```python
from build123d import *

# Parameters (mm, degrees)
BOSS_EXTRUDE1_DEPTH = 3
SKETCH2_R           = 1.55
CUT_EXTRUDE1_DEPTH  = 356.878676658
BOSS_EXTRUDE3_START = -6
SKETCH3_R           = 1.55
BOSS_EXTRUDE3_DEPTH = 6


with BuildPart() as part:
    # Sketch1 → Boss-Extrude1 (new body)
    with BuildSketch(Plane(origin=(0, 0, 0), x_dir=(1, 0, 0), z_dir=(0, 1, 0))):
        Polygon((5.02071, 249.35), (4.05, 248.379), (4.05, 235), (4.04962, 234.998), (4.04981, 234.996), (4.04812, 234.989), (4.04698, 234.983), (4.04588, 234.981), (4.04531, 234.979), (4.04157, 234.974), (4.0383, 234.968), (4.03662, 234.966), (4.03536, 234.965), (0.095609, 231.025), (0.1, 231), (0.1, 10.0414), (25.0414, -14.9), (36.9586, -14.9), (42.9293, -8.92929), (42.9329, -8.92677), (42.9357, -8.9234), (42.947, -8.91686), (42.9577, -8.90937), (42.962, -8.90823), (42.9658, -8.90603), (42.9787, -8.90376), (42.9913, -8.90038), (42.9957, -8.90076), (43, -8.9), (211, -8.9), (211.004, -8.90076), (211.009, -8.90038), (211.021, -8.90376), (211.034, -8.90603), (211.038, -8.90823), (211.042, -8.90937), (211.053, -8.91687), (211.064, -8.9234), (211.067, -8.92676), (211.071, -8.92929), (217.041, -14.9), (228.959, -14.9), (253.9, 10.0414), (253.9, 230.959), (249.959, 234.9), (209, 234.9), (208.966, 234.906), (208.936, 234.923), (208.913, 234.95), (208.902, 234.983), (208.902, 235.017), (208.904, 235.025), (202.979, 240.95), (191.021, 240.95), (185.096, 235.025), (185.098, 235.017), (185.098, 234.983), (185.087, 234.95), (185.064, 234.923), (185.034, 234.906), (185, 234.9), (69, 234.9), (68.9658, 234.906), (68.9357, 234.923), (68.9134, 234.95), (68.9015, 234.983), (68.9015, 235.017), (68.9043, 235.025), (62.9793, 240.95), (51.0207, 240.95), (45.0957, 235.025), (45.0985, 235.017), (45.0985, 234.983), (45.0866, 234.95), (45.0643, 234.923), (45.0342, 234.906), (45, 234.9), (34, 234.9), (33.9658, 234.906), (33.9357, 234.923), (33.9134, 234.95), (33.9015, 234.983), (33.9015, 235.017), (33.9043, 235.025), (32.9646, 235.965), (32.9634, 235.966), (32.9617, 235.968), (32.9584, 235.974), (32.9547, 235.979), (32.9541, 235.981), (32.953, 235.983), (32.9519, 235.989), (32.9502, 235.996), (32.9504, 235.998), (32.95, 236), (32.95, 248.379), (31.9793, 249.35), align=None)
    extrude(amount=BOSS_EXTRUDE1_DEPTH)

    # Sketch2 → Cut-Extrude1 (cut, through all)
    with BuildSketch(Plane(origin=(0, 3, 0), x_dir=(1, 0, 0), z_dir=(0, 1, 0))):
        with Locations(Location((17, 10.0414, 0), (0, 0, 270))):
            Circle(SKETCH2_R)
        with Locations(Location((127, 10.0414, 0), (0, 0, 270))):
            Circle(SKETCH2_R)
        with Locations(Location((232, 10.0414, 0), (0, 0, 270))):
            Circle(SKETCH2_R)
        with Locations(Location((232, 115.0414, 0), (0, 0, 270))):
            Circle(SKETCH2_R)
        with Locations(Location((232, 220.0414, 0), (0, 0, 270))):
            Circle(SKETCH2_R)
        with Locations(Location((127, 115.0414, 0), (0, 0, 270))):
            Circle(SKETCH2_R)
        with Locations(Location((17, 115.0414, 0), (0, 0, 270))):
            Circle(SKETCH2_R)
        with Locations(Location((17, 220.0414, 0), (0, 0, 270))):
            Circle(SKETCH2_R)
        with Locations(Location((127, 220.0414, 0), (0, 0, 270))):
            Circle(SKETCH2_R)
        with Locations(Location((197, 231, 0), (0, 0, 270))):
            Circle(SKETCH2_R)
        with Locations(Location((57, 231, 0), (0, 0, 270))):
            Circle(SKETCH2_R)
        with Locations(Location((18.499978099, 242, 0), (0, 0, 270))):
            Circle(SKETCH2_R)
    extrude(amount=-CUT_EXTRUDE1_DEPTH, mode=Mode.SUBTRACT)

    # Sketch3 → Boss-Extrude3 (add)
    with BuildSketch(Plane.XZ.offset(BOSS_EXTRUDE3_START)):
        with Locations(Location((57, -231, 0), (0, 0, 270))):
            Circle(SKETCH3_R)
        with Locations(Location((197, -231, 0), (0, 0, 270))):
            Circle(SKETCH3_R)
    extrude(amount=BOSS_EXTRUDE3_DEPTH)


solid = part.part
```
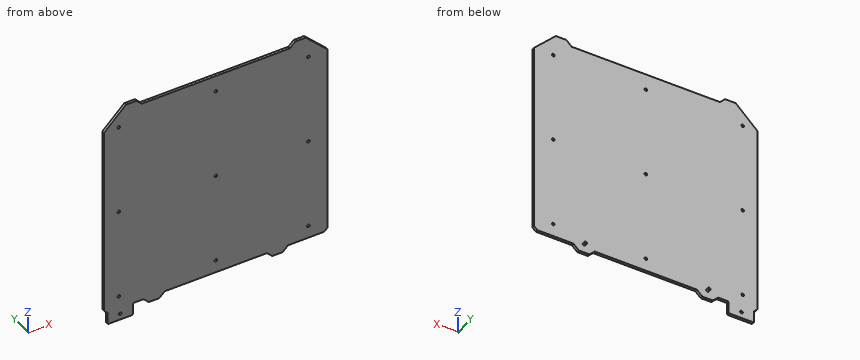
Geometry check sheet. Reference: the model listing, model coordinates, mm. Give positions to 0.01 mm unless a question says otherwise; leave off trailing zeros. Order: outer loops, then holes, each group sorted by start corner. A loop starts at its lowest first (then second) coordinate and runs counter-clockwise, first axis right, second up.
1. Gauge pin test, flat ends, axial feed: pin 1 Ø2.5 at (x, z) = (232, -220.04) entering from -Y; pin 2 Ø3.5 at (x, y) = (37, 1) entering from -Z; pin 3 Ø1.5 at (x, y) = (68, 1) entering from -Z; pin 4 Ø3.5 at (x, z) = (127, -115.04) entering from +Y. Record the tip position at first contact, or that the pin passes through.
2. Section check C-C, the plane y = 0.95. Give the number of separate pieces and of enclosed holes in the cut face, and give its area (3 significant figures).
3. Section check A-A, the plane z = -201. Enter the section's corners in (x, y), and give its area (3 significant figures).
4. Thickness scan on L1, parallel to Z at x = 127, y = 1.5; L2, parallel to Z at x = 232, y = 1.3; L3, parallel to X at y = 0.55, z = -224.5. Record the ranges inside material, lowest first.
5. Section check B-B, the plane x = 96. Enter the section's corners in (y, z).
Values follow:
1. pin 1: passes through
1. pin 2: stops at z = -234.9
1. pin 3: stops at z = -236.68
1. pin 4: stops at y = 3
2. separate pieces: 1
2. enclosed holes: 10
2. area: 62,300 mm2
3. outline: (0.1, 0) - (253.9, 0) - (253.9, 3) - (0.1, 3) - close
3. area: 761 mm2
4. L1: z = -234.9 to -221.59, -218.49 to -116.59, -113.49 to -11.59, -8.49 to 8.9
4. L2: z = -234.9 to -221.59, -218.49 to -116.59, -113.49 to -11.59, -8.49 to 11.86
4. L3: x = 0.1 to 253.9
5. outline: (0, -234.9) - (3, -234.9) - (3, 8.9) - (0, 8.9) - close
